Autodesk Inventor part; units mm, degrees
ref_plane "YZ Plane" through (0, 0, 0) normal (1, 0, 0) x (0, 1, 0)
ref_plane "XZ Plane" through (0, 0, 0) normal (0, 1, 0) x (-1, 0, 0)
ref_plane "XY Plane" through (0, 0, 0) normal (0, 0, 1) x (1, 0, 0)
sketch "Sketch1" plane through (0, 0, 0) normal (0, 1, 0) x (-1, 0, 0)
  circle A0 centre (0, 0) radius 6.75
  circle A1 centre (0, 0) radius 6.25
  dimension "d0" = 13.5
  dimension "d1" = 12.5
extrude "Extrusion1" add sketch "Sketch1" along normal blind 30
sketch "Sketch8" plane through (0, 0, 0) normal (0, -1, 0) x (1, 0, 0)
  circle A0 centre (0, 0) radius 6.25
  circle A1 centre (0, 0) radius 3.875
  dimension "d32" = 7.75
extrude "Extrusion8" add sketch "Sketch8" against normal blind 3
chamfer "Chamfer2" distance 0.1 distance2 2 1 edges at (-3.875, 0, 0) measured on face at (-5.6888, 0, -0.8476)
sketch "Sketch9" plane through (0, 0, 0) normal (0, -1, 0) x (1, 0, 0)
  circle A0 centre (0, 0) radius 3.975
  line L0 (10, -10) -> (-10, -10)
  line L1 (-10, -10) -> (-10, 10)
  line L2 (-10, 10) -> (10, 10)
  line L3 (10, 10) -> (10, -10)
  line L4 (10, -10) -> (-10, 10) construction
  line L5 (-10, -10) -> (10, 10) construction
  dimension "d38" = 20
  dimension "d39" = 20
extrude "Extrusion9" add sketch "Sketch9" along normal blind 3
ref_plane "Work Plane1" through (0, -3, 10) normal (1, 0, 0) x (0, 0, -1)
properties part number "MOULD"
The listing builds one solid part. Answer for the finished solid, in the listing's coordinates (mm). A direction names the side the tool comes from. Give positions to 0.01 mm unless a question says otherwise; leave off trailing zeros. Order: outer loops, then holes, each group sorted by start corner. A loop starts at its lowest first (then second) coordinate and runs counter-clockwise, first axis right, second up. Notation, with made-up numbers: (13, 16.5) - (19, 16.5) arc R11 ccw to (19, 22.5) - close; hole circle Ø6 at (78, -16). An arc over 180 degrees is marked (long way). One line per item, written item: value. Start each with the question number.
1) A cutting plane is placed at D-D on z = -8. Give the vertices of the cut face in (x, y), then the cut area to 3 significant figures.
2) A cutting plane is placed at B-B on x = 0. Give the vertices of the cut face in (y, z) (3 decimals).
3) Find the intervals of material crossed by L1, parallel to Z at x = 0, y = 2.85 (3 decimals); L2, parallel to Z at x = 0, y = 9; L3, parallel to Y at x = 6.5, z = 6, in increasing order.
4) A cutting plane is placed at A-A on z = 0. Give the vertices of the cut face in (x, y) (3 decimals).
5) A tool of negligible diameter and unlimited length cuts with its end or side. For faces 4 (the face through (-5.96, 16.31, -1.88)), 5 (the face through (10, -1, 0)), from which of +Z, -Z, +X, -X, +Y, -Y can it reach the whole face along a straight path? Write none if from no direction.
6) The mould has two halves that part along X. Classify faces 1 (the face through (-7, 0, 0)), 2 (the face through (-10, -1, 0)), 3 (the face through (-0.86, -1.48, 3.88)): released by +X, released by -X, zero draft, split by the parting line, or undercut.
7) A cutting plane is placed at C-C on y = 18.5. Give the vertices of the cut face in (x, z).
8) Given pin 1 Ø6 at (x, y) = (-7, 22) entering from -Z; pin 2 Ø4 at (y, z) = (3, 1.5) entering from -X; pin 3 Ø9 at (x, z) = (0, 0) entering from +Y, each flat-ended and moving along its own axis, determine where each tip first touches the part or whether it passes through.
Answer sheet:
1. outline: (-10, -3) - (10, -3) - (10, 0) - (-10, 0) - close
1. area: 60.0 mm2
2. outline: (-3, -10) - (0, -10) - (0, -6.75) - (30, -6.75) - (30, -6.25) - (3, -6.25) - (3, -3.875) - (2, -3.875) - (0, -3.975) - (-3, -3.975) - close; (-3, 3.975) - (0, 3.975) - (2, 3.875) - (3, 3.875) - (3, 6.25) - (30, 6.25) - (30, 6.75) - (0, 6.75) - (0, 10) - (-3, 10) - close
3. L1: z = -6.75 to -3.875, 3.875 to 6.75
3. L2: z = -6.75 to -6.25, 6.25 to 6.75
3. L3: y = -3 to 0
4. outline: (-10, -3) - (-3.975, -3) - (-3.975, 0) - (-3.875, 2) - (-3.875, 3) - (-6.25, 3) - (-6.25, 30) - (-6.75, 30) - (-6.75, 0) - (-10, 0) - close; (3.875, 2) - (3.975, 0) - (3.975, -3) - (10, -3) - (10, 0) - (6.75, 0) - (6.75, 30) - (6.25, 30) - (6.25, 3) - (3.875, 3) - close
5. face 4: +Y
5. face 5: +Z, -Z, +X, +Y, -Y
6. face 1: zero draft
6. face 2: released by -X
6. face 3: undercut
7. outline: circle Ø13.5 at (0, 0); hole circle Ø12.5 at (0, 0)
8. pin 1: stops at z = -5.44
8. pin 2: stops at x = -6.75
8. pin 3: stops at y = 3
